For this review, take the finished solid that the model builds, in its own axes (mm). A direction names the side the tool comes from. Coordinates: 2 decimals unless noted, no trailing zeros. Write each loop counter-clockwise with the first axis right and the second up, starting at its lowest first coordinate (ties: lowest second). Pieces come first, ordered by that corner, then holes. Notation, with made-up numbers: (-30, -23.75) - (4, -23.75) arc R19 cw to (4, -2.75) - close; hole circle Ø5 at (12, 19.25). An arc over 180 degrees is marked (long way). Use one line per item in the form item = value. Start each with the question number.
1) Tool access review of faces 3 (the flat face through (-30.25, 0, 9)), 4 (the flat face through (-34, 0, 10.5)): name each direction out of +Z, -Z, +X, -X, +Y, -Y from which nothing blocks a thin tool from reaching the whole face with its end or side.
2) We need section D-D (x = -23.5). Count the separate pieces of the cut face and the enclosed holes in it, plus the area to 3 significant figures.
3) Insertion check: P1, Ø5, axis at y = 22.5, z = 5.5, coming from the +X side; P2, Ø6.5, axis at x = -24.04, y = -24.04, coming from the +Z side; P3, Ø2.5, axis at x = 12, z = 9.5, coming from the +Y side. Each pin has a flat end and moves straight along its axis. Give the tip position at first contact, or say it passes through.
4) We need section C-C (z = 1.25). Give the boundary of the cut face in (x, y), plus the area to 3 significant figures.
5) We need section A-A (y = 0). Give the boundary of the cut face in (x, z) (3 decimals), plus the area to 3 significant figures.
6) Mouldability with a two-part tool opening along Y and no side actions: class faces 1 (the flat face through (0, -34, 10.5)), 2 (the flat face through (30.25, 0, 9)) as pulls with the +Y half, pulls with the -Y half, needs draft (parallel to the pull), parting line crosses it, or undercut.
7) For L1, parallel to X at y = 25.5, z = 3; L2, parallel to Y at x = -1, z = 9.25; L3, parallel to X at y = 22.5, z = 7, list the stretches that pass through material, from the lowest coordinate up. Write a range as from..to.
```python
from build123d import *

# Parameters (mm, degrees)
SKETCH2_R           = 2.5
CUT_EXTRUDE2_DEPTH  = 58.534772252
BOSS_EXTRUDE1_START = -10.5
BOSS_EXTRUDE1_DEPTH = 10.5


with BuildPart() as part:
    # Sketch1 → Revolve1 (revolve)
    with BuildSketch(Plane(origin=(0, 0, 0), x_dir=(1, 0, 0), z_dir=(0, 1, 0)), mode=Mode.PRIVATE) as revolve1_sk:
        with BuildLine():
            Line((29.5, 0), (40, 0))
            Line((40, 0), (40, -10.5))
            ThreePointArc((40, -10.5), (35.334867618, -9.033526194), (30.5, -8.3))
            Line((30.5, -8.3), (29.5, -5))
            Line((29.5, -5), (29.5, 0))
        make_face()
    revolve(revolve1_sk.sketch.rotate(Axis((0, 0, 0), (0, 0, 1)), 180), axis=Axis((0, 0, 0), (0, 0, 1)))

    # Sketch2 → Cut-Extrude2 (cut, through all)
    with BuildSketch(Plane(origin=(0, 0, 0), x_dir=(-1, 0, 0), z_dir=(0, 0, -1))):
        with Locations((24.04163056, 24.04163056)):
            Circle(SKETCH2_R)
        with Locations((24.04163056, -24.04163056)):
            Circle(SKETCH2_R)
        with Locations((-24.04163056, -24.04163056)):
            Circle(SKETCH2_R)
        with Locations((-24.04163056, 24.04163056)):
            Circle(SKETCH2_R)
    extrude(amount=-CUT_EXTRUDE2_DEPTH, mode=Mode.SUBTRACT)

    # Sketch4 → Boss-Extrude1 (add)
    with BuildSketch(Plane(origin=(0, 0, 0), x_dir=(-1, 0, 0), z_dir=(0, 0, -1)).offset(BOSS_EXTRUDE1_START)):
        with BuildLine():
            Line((-26.171310628, 30.25), (26.171310628, 30.25))
            ThreePointArc((26.171310628, 30.25), (0, 40), (-26.171310628, 30.25))
        make_face()
        with BuildLine():
            Line((-30.25, 26.171310628), (-30.25, -26.171310628))
            ThreePointArc((-30.25, -26.171310628), (-40, 0), (-30.25, 26.171310628))
        make_face()
        with BuildLine():
            Line((-26.171310628, -30.25), (26.171310628, -30.25))
            ThreePointArc((26.171310628, -30.25), (0, -40), (-26.171310628, -30.25))
        make_face()
        with BuildLine():
            Line((30.25, 26.171310628), (30.25, -26.171310628))
            ThreePointArc((30.25, -26.171310628), (40, 0), (30.25, 26.171310628))
        make_face()
    extrude(amount=BOSS_EXTRUDE1_DEPTH)


solid = part.part
```
Determined:
q1.face_3 = +Z
q1.face_4 = +Z, +X, -X, +Y, -Y
q2.separate_pieces = 4
q2.enclosed_holes = 0
q2.area = 173 mm²
q3.P1 = 34.64
q3.P2 = 9.54
q3.P3 = 38.53
q4.outline = circle Ø80 at (0, 0); hole circle Ø59 at (0, 0); hole circle Ø5 at (-24.04, -24.04); hole circle Ø5 at (-24.04, 24.04); hole circle Ø5 at (24.04, -24.04); hole circle Ø5 at (24.04, 24.04)
q4.area = 2,210 mm²
q5.outline = (-40, 0) - (-29.5, 0) - (-29.5, 5) - (-30.25, 7.475) - (-30.25, 10.5) - (-40, 10.5) - close; (29.5, 0) - (40, 0) - (40, 10.5) - (30.25, 10.5) - (30.25, 7.475) - (29.5, 5) - close
q5.area = 214 mm²
q6.face_1 = needs draft
q6.face_2 = undercut
q7.L1 = -30.82..-26.07, -22.01..-14.83, 14.83..22.01, 26.07..30.82
q7.L2 = -39.99..-30.25, 30.25..39.99
q7.L3 = -33.07..-26.01, -22.07..-20, 20..22.07, 26.01..33.07
